Check sheet for the modelled part. Datum: model origin and axes. Units: mm. Face numbers are marked on the shaded views. A direction names the side the tool comes from. Give positions to 0.01 mm unless a question says otherwise; leave off trailing zeros. Loops run counter-clockwise (first coordinate to the right, second up) from the corner with the lowest first, then second, coordinate; pieces in that order, holes last. Notation, with made-up numbers: (-11.75, 26.25) - (13.25, 26.25) arc R4 cw to (13.25, 32.25) - close; hole circle Ø5 at (16.5, 32). An arc over 180 degrees is marked (long way). Use CSV: the item, a comma, the result in double quotes.
from build123d import *

# Parameters (mm, degrees)
SKETCH_1_W          = 20
SKETCH_1_H          = 20
EXTRUDE_1_DEPTH     = 20
SKETCH_3_W          = 10
SKETCH_3_H          = 10
CUT_EXTRUDE_1_DEPTH = 20
SKETCH_4_W          = 20
SKETCH_4_H          = 32
EXTRUDE_2_DEPTH     = 15
SKETCH_5_W          = 20
SKETCH_5_H          = 22
CUT_EXTRUDE_2_DEPTH = 10


with BuildPart() as part:
    # 草图1 → 凸台-拉伸1 (new body)
    with BuildSketch(Plane.XY):
        with Locations((10, 10)):
            Rectangle(SKETCH_1_W, SKETCH_1_H)
    extrude(amount=EXTRUDE_1_DEPTH)

    # 草图3 → 切除-拉伸1 (cut)
    with BuildSketch(Plane(origin=(0, 0, 0), x_dir=(-1, 0, 0), z_dir=(0, 0, -1))):
        with Locations((-10, 10)):
            Rectangle(SKETCH_3_W, SKETCH_3_H)
    extrude(amount=-CUT_EXTRUDE_1_DEPTH, mode=Mode.SUBTRACT)

    # 草图4 → 凸台-拉伸2 (add)
    with BuildSketch(Plane(origin=(0, 0, 0), x_dir=(-1, 0, 0), z_dir=(0, 0, -1))):
        with Locations((-10, 10)):
            Rectangle(SKETCH_4_W, SKETCH_4_H)
    extrude(amount=EXTRUDE_2_DEPTH)

    # 草图5 → 切除-拉伸2 (cut)
    with BuildSketch(Plane(origin=(0, 0, -15), x_dir=(-1, 0, 0), z_dir=(0, 0, -1))):
        with Locations((-10, 10)):
            Rectangle(SKETCH_5_W, SKETCH_5_H)
    extrude(amount=-CUT_EXTRUDE_2_DEPTH, mode=Mode.SUBTRACT)


solid = part.part
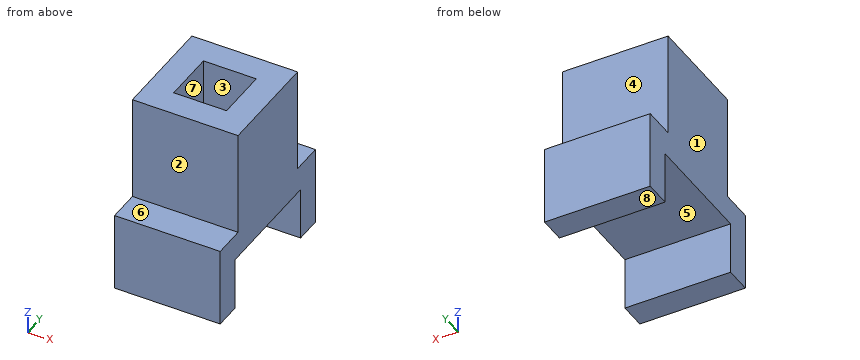
1. Sectioned sample at A-A, the plane z = -11.5. Record the boundary of the cut face in (x, y), and give its area (3 significant figures).
Completed:
outline,"(0, -6) - (20, -6) - (20, -1) - (0, -1) - close; (0, 21) - (20, 21) - (20, 26) - (0, 26) - close"
area,"200 mm²"
2. Set-up check for the marked faces 4, 5, 6, 7 and 8: record each of +Z, -Z, +X, -X, +Y, -Y from which the full face is reachable in a straight line by a thin tool's end or side.
Completed:
face 4,"+Z, +X, -X, +Y"
face 5,"-Z, +X, -X"
face 6,"+Z, +X, -X, -Y"
face 7,"+Z"
face 8,"-Z, +X, -X, +Y, -Y"
3. Sectioned sample at D-D, the plane y = -4. Record the boundary of the cut face in (x, z).
Completed:
outline,"(0, -15) - (20, -15) - (20, 0) - (0, 0) - close"
4. Sectioned sample at C-C, the plane x = 7.5. Record the boundary of the cut face in (y, z), and give its area (3 significant figures).
Completed:
outline,"(-6, -15) - (-1, -15) - (-1, -5) - (21, -5) - (21, -15) - (26, -15) - (26, 0) - (20, 0) - (20, 20) - (15, 20) - (15, 0) - (5, 0) - (5, 20) - (0, 20) - (0, 0) - (-6, 0) - close"
area,"460 mm²"
5. Go/stop test with flat-tipped pins: pin 1 Ø10 at (x, y) = (5.5, 14) entering from -Z; pin 2 Ø3 at (x, y) = (9.5, 11.5) entering from +Z; pin 3 Ø4 at (x, z) = (11, 15) entering from +Y. Record where each tip stops, or that it passes through.
Completed:
pin 1,"stops at z = -5"
pin 2,"stops at z = 0"
pin 3,"stops at y = 20"
6. Sectioned sample at B-B, the plane z = 6. Record the boundary of the cut face in (x, y).
Completed:
outline,"(0, 0) - (20, 0) - (20, 20) - (0, 20) - close; hole (5, 5) - (15, 5) - (15, 15) - (5, 15) - close"
7. Release check for a two-part mould opening along X. For the marked faces 1, 2 and 3 record: released by +X, released by -X, zero draft, split by the parting line, or undercut.
Completed:
face 1,"released by -X"
face 2,"zero draft"
face 3,"undercut"
8. Scan lines: line 1 along Y through (x, z) = (10.25, 9); line 2 along Z through (x, y) = (11, 3). Record each from-to range of solid material in increasing order.
Completed:
line 1,"y = 0 to 5, 15 to 20"
line 2,"z = -5 to 20"
